Autodesk Inventor part; units mm, degrees
ref_plane "YZ Plane" through (0, 0, 0) normal (1, 0, 0) x (0, 1, 0)
ref_plane "XZ Plane" through (0, 0, 0) normal (0, 1, 0) x (-1, 0, 0)
ref_plane "XY Plane" through (0, 0, 0) normal (0, 0, 1) x (1, 0, 0)
sketch "Sketch1" plane through (0, 0, 0) normal (0, 0, 1) x (1, 0, 0)
  circle A0 centre (0, 0) radius 30
  line L0 (0, 0) -> (20, 0)
  line L1 (20, 0) -> (20, 150)
  line L2 (20, 150) -> (0, 150)
  line L3 (0, 150) -> (0, 0)
  line L4 (0, 0) -> (-20, 0)
  line L5 (-20, 0) -> (-20, 150)
  line L6 (-20, 150) -> (0, 150)
  line L7 (0, 150) -> (0, 0)
  circle A1 centre (0, 150) radius 30
  point P0 (20, 127.6393)
  point P1 (-20, 127.6393)
  point P2 (-20, 22.3607)
  point P3 (20, 22.3607)
  dimension "d0" = 60
  dimension "d1" = 20
  dimension "d2" = 150
  dimension "d3" = 20
  dimension "d4" = 60
extrude "Extrusion1" add sketch "Sketch1" along normal blind 20
sketch "Sketch2" plane through (0, 0, 20) normal (0, 0, 1) x (1, 0, 0)
  circle A0 centre (0, 0) radius 10
  dimension "d7" = 20
extrude "Extrusion2" cut sketch "Sketch2" against normal blind 16
sketch "Sketch3" plane through (0, 0, 4) normal (0, 0, 1) x (1, 0, 0)
  circle A0 centre (0, 0) radius 1.5
  circle A1 centre (-7, 0) radius 1.5
  circle A2 centre (7, 0) radius 1.5
  dimension "d10" = 3
  dimension "d11" = 3
  dimension "d12" = 3
extrude "Extrusion3" cut sketch "Sketch3" against normal blind 25.275
sketch "Sketch4" plane through (0, 0, 20) normal (0, 0, 1) x (1, 0, 0)
  circle A0 centre (0, 150) radius 10
  line L0 (-10, 150) -> (10, 150)
  line L1 (10, 150) -> (10, 110)
  line L2 (10, 110) -> (-10, 110)
  line L3 (-10, 110) -> (-10, 150)
  circle A1 centre (0, 150) radius 6
  line L4 (-6, 150) -> (6, 150)
  line L5 (6, 150) -> (6, 127)
  line L6 (6, 127) -> (-6, 127)
  line L7 (-6, 127) -> (-6, 150)
  line L8 (-6, 150) -> (6, 150)
  line L9 (6, 150) -> (6, 156)
  line L10 (6, 156) -> (-6, 156)
  line L11 (-6, 156) -> (-6, 150)
  point P0 (0, 0)
  dimension "d15" = 20
  dimension "d17" = 12
  dimension "d16" = 40
  dimension "d18" = 23
extrude "Extrusion4" cut sketch "Sketch4" against normal blind 13 contours L5 L6 L7 A0 | A0 L7 A1 L5 | A1 L0 | L0 A1 | A1 L10 L9 | L11 L10 A1
sketch "Sketch5" plane through (0, 0, 20) normal (0, 0, 1) x (1, 0, 0)
  line L0 (6, 127) -> (-6, 127)
  line L1 (-6, 127) -> (6, 127)
  line L2 (6, 127) -> (6, 122.3)
  line L3 (6, 122.3) -> (-6, 122.3)
  line L4 (-6, 122.3) -> (-6, 127)
  line L5 (-6, 156) -> (6, 156)
  line L6 (-6, 156) -> (6, 156)
  line L7 (6, 156) -> (6, 160.7)
  line L8 (6, 160.7) -> (-6, 160.7)
  line L9 (-6, 160.7) -> (-6, 156)
  point P0 (0, 0)
  dimension "d21" = 4.7
  dimension "d22" = 4.7
extrude "Extrusion5" cut sketch "Sketch5" against normal blind 11.5
sketch "Sketch6" plane through (0, 0, 8.5) normal (0, 0, 1) x (1, 0, 0)
  line L0 (-6, 160.7) -> (6, 160.7)
  line L1 (6, 160.7) -> (6, 156)
  line L2 (-6, 160.7) -> (6, 160.7)
  line L3 (6, 160.7) -> (6, 158.4)
  line L4 (6, 158.4) -> (-6, 158.4)
  line L5 (-6, 158.4) -> (-6, 160.7)
  circle A0 centre (0, 158.4) radius 1
  line L6 (-6, 122.3) -> (-6, 127)
  line L7 (6, 127) -> (6, 122.3)
  line L8 (-6, 122.3) -> (6, 122.3)
  line L9 (6, 122.3) -> (6, 124.6)
  line L10 (6, 124.6) -> (-6, 124.6)
  line L11 (-6, 124.6) -> (-6, 122.3)
  circle A1 centre (0, 124.6) radius 1
  point P0 (0, 0)
  dimension "d25" = 2.3
  dimension "d26" = 2
  dimension "d27" = 2.3
  dimension "d28" = 2
extrude "Extrusion6" cut sketch "Sketch6" against normal blind 5 contours A0 L4 | L4 A0 | A1 L10 | L10 A1
sketch "Sketch7" plane through (0, 0, 0) normal (0, 0, -1) x (-1, 0, 0)
  circle A0 centre (0, 150) radius 10
  point P0 (0, 0)
  dimension "d31" = 20
extrude "Extrusion7" cut sketch "Sketch7" against normal blind 8
chamfer "Chamfer1" distance 16 angle 45 1 edges at (-10, 0, 20)
sketch "Sketch8" plane through (0, 0, 20) normal (0, 0, 1) x (1, 0, 0)
  arc A0 (20, 127.6393) -> (-20, 127.6393) centre (0, 150) ccw
  line L0 (-20, 127.6393) -> (-20, 22.3607)
  line L1 (20, 127.6393) -> (-20, 22.3607)
  line L2 (-20, 22.3607) -> (-20, 127.6393)
  line L3 (20, 22.3607) -> (20, 127.6393)
  line L4 (-20, 127.6393) -> (20, 22.3607)
  line L5 (20, 127.6393) -> (20, 22.3607)
  line L6 (0, 75) -> (8.2239, 75)
  line L7 (8.2239, 75) -> (8.2239, 53.3549)
  line L8 (8.2239, 53.3549) -> (0, 53.3549)
  line L9 (0, 53.3549) -> (0, 75)
  line L10 (0, 75) -> (-8.2239, 75)
  line L11 (-8.2239, 75) -> (-8.2239, 53.3549)
  line L12 (-8.2239, 53.3549) -> (0, 53.3549)
  line L13 (0, 53.3549) -> (0, 75)
  line L14 (8.2239, 75) -> (-8.2239, 75)
  line L15 (-8.2239, 75) -> (-8.2239, 96.6451)
  line L16 (-8.2239, 96.6451) -> (8.2239, 96.6451)
  line L17 (8.2239, 96.6451) -> (8.2239, 75)
  point P0 (0, 0)
extrude "Extrusion8" cut sketch "Sketch8" against normal blind 64.1375 contours L3 L4 L7 L17 L1 | L4 L15 L11 L1 L0
properties part number "1st-arm"
For this review, take the finished solid that the model builds, in its own axes (mm). A direction names the side the tool comes from. Give positions to 0.01 mm unless a question says otherwise; leave off trailing zeros. Loops run counter-clockwise (first coordinate to the right, second up) from the corner with the lowest first, then second, coordinate; pieces in that order, holes last. Notation, with made-up numbers: M -6,-28.75 L 52,-28.75 A8 cw 52,-21.75 Z; hole C -1,-22 d10. An arc over 180 degrees is marked long. Put each result on its own line as item: value. Start each with the question number.
(1) Wall thickness on L1, parallel to Y at x = 0, z = 2; L2, parallel to Y at x = 0, z = 8.3; L3, parallel to Y at x = 2.5, z = 16.75: over which ranges is each line inside the solid? List them lowest first.
(2) Add section A-A, the plane y = 150. Write out the cut boundary in (x, z).
(3) Add section B-B, the plane z = 16. Give the number of separate pieces and of enclosed holes in the cut face, then the cut area to 3 significant figures.
(4) For pin 1 (1.5 mm diameter, centred on x = 4, z = 16.5, fed in from +Y); pin 2 (6 mm diameter, centred on x = 1.5, y = 133.5, fed in from +Z); pin 3 (8 mm diameter, centred on x = 3.5, z = 12.5, fed in from +Y); pin 4 (1.5 mm diameter, centred on x = -22, y = 128, fed in from -Z), all flat-tipped, find the tip position at first contact; note any pin that passes through.
(5) Machinability: for faces 3 (the flat face through (-14.194, 112.359, 10.14)), 4 (the flat face through (0, 135, 7)), 5 (the flat face through (0, 157, 8)), 6 (the flat face through (8.224, 75, 10)), which of the approach directions +Z, -Z, +X, -X, +Y, -Y give a long, thin tool a straight path to every point of the face, cutting with its end or side? Answer none if there is none.
(6) The part is to be moulded in two halves that separate along Y. For faces 1 (the flat face through (0, 100, 20)), 2 (the flat face through (-8.224, 75, 10)), say which applies: +Y half, -Y half, draft (parallel to the pull), parting line (faces both ways), or undercut.
(7) Add section C-C, the plane y = 108.5. Write out the cut boundary in (x, z), then the cut area to 3 significant figures.
Result:
1. L1: y = -30 to -1.5, 1.5 to 140, 160 to 180
1. L2: y = -30 to -14.3, 14.3 to 123.6, 125.6 to 127, 156 to 157.4, 159.4 to 180
1. L3: y = -29.9 to -22.61, 22.61 to 122.3, 160.7 to 179.9
2. outline: M -30,0 L -10,0 L -10,8 L -6,8 L -6,20 L -30,20 Z; M 6,8 L 10,8 L 10,0 L 30,0 L 30,20 L 6,20 Z
3. separate pieces: 1
3. enclosed holes: 2
3. area: 5,720 mm^2
4. pin 1: stops at y = 179.82
4. pin 2: stops at z = 7
4. pin 3: stops at y = 180
4. pin 4: passes through
5. face 3: +Z, -Z, -X
5. face 4: +Z
5. face 5: -Z
5. face 6: +Z, -Z, +X
6. face 1: draft
6. face 2: undercut
7. outline: M -12.73,0 L 12.73,0 L 12.73,20 L -12.73,20 Z
7. area: 509 mm^2
